Autodesk Inventor part; units mm, degrees
ref_plane "YZ Plane" through (0, 0, 0) normal (1, 0, 0) x (0, 1, 0)
ref_plane "XZ Plane" through (0, 0, 0) normal (0, 1, 0) x (-1, 0, 0)
ref_plane "XY Plane" through (0, 0, 0) normal (0, 0, 1) x (1, 0, 0)
sketch "Sketch2" plane through (0, 0, 0) normal (0, 0, 1) x (1, 0, 0)
  line L0 (-50.1541, 26.4593) -> (-15.1541, 26.4593)
  line L1 (-15.1541, 26.4593) -> (-15.1541, 29.4593)
  line L2 (-15.1541, 29.4593) -> (34.8459, 29.4593)
  line L3 (34.8459, 29.4593) -> (34.8459, 26.4593)
  line L4 (34.8459, 26.4593) -> (69.8459, 26.4593)
  line L5 (-50.1541, 26.4593) -> (-50.1541, -70.5407)
  line L6 (-50.1541, -70.5407) -> (-15.1541, -70.5407)
  line L7 (-15.1541, -70.5407) -> (-15.1541, -73.5407)
  line L8 (-15.1541, -73.5407) -> (34.8459, -73.5407)
  line L9 (34.8459, -73.5407) -> (34.8459, -70.5407)
  line L10 (34.8459, -70.5407) -> (69.8459, -70.5407)
  line L11 (69.8459, -70.5407) -> (69.8459, 26.4593)
  point P0 (0, 0)
  dimension "d0" = 3
  dimension "d1" = 50
  dimension "d2" = 35
  dimension "d3" = 35
  dimension "d4" = 97
  dimension "d5" = 97
  dimension "d6" = 3
  dimension "d7" = 35
  dimension "d8" = 50
  dimension "d9" = 35
extrude "Extrusion1" add sketch "Sketch2" along normal blind 3
sketch "Sketch3" plane through (0, 0, 3) normal (0, 0, 1) x (1, 0, 0)
  line L0 (34.8459, 29.4593) -> (-15.1541, 29.4593)
  line L1 (-15.1541, -73.5407) -> (34.8459, -73.5407)
  line L2 (-50.1541, 26.4593) -> (-50.1541, -70.5407)
  line L3 (69.8459, -70.5407) -> (69.8459, 26.4593)
  circle A0 centre (57.6459, 1.2193) radius 2
  circle A1 centre (57.6459, -45.5807) radius 2
  circle A2 centre (-28.3541, 1.2193) radius 2
  circle A3 centre (-28.3541, -45.5807) radius 2
  circle A4 centre (47.3959, -22.1807) radius 7
  line L4 (-16.4541, -2.7807) -> (34.4459, -2.7807)
  line L5 (34.4459, -2.7807) -> (34.4459, -42.7807)
  line L6 (34.4459, -42.7807) -> (-16.4541, -42.7807)
  line L7 (-16.4541, -42.7807) -> (-16.4541, -2.7807)
  line L8 (-38.3241, -7.0307) -> (-31.4241, -7.0307)
  line L9 (-31.4241, -7.0307) -> (-31.4241, -37.4307)
  line L10 (-31.4241, -37.4307) -> (-38.3241, -37.4307)
  line L11 (-38.3241, -37.4307) -> (-38.3241, -7.0307)
  point P0 (0, 0)
  dimension "d30" = 4
  dimension "d34" = 4
  dimension "d35" = 4
  dimension "d36" = 4
  dimension "d38" = 14
  dimension "d43" = 50.9
  dimension "d44" = 40
extrude "Extrusion2" cut sketch "Sketch3" against normal blind 10
sketch "Sketch4" plane through (-38.3241, -37.4307, 3) normal (1, 0, 0) x (0, 0, -1)
  line L0 (0, 30.4) -> (3, 30.4)
  line L1 (3, 30.4) -> (3, 0)
  line L2 (3, 0) -> (0, 0)
  line L3 (0, 0) -> (0, 30.4)
  point P0 (3, 37.4307)
extrude "Extrusion3" add sketch "Sketch4" along normal blind 10
sketch "Sketch5" plane through (0, 0, 3) normal (0, 0, 1) x (1, 0, 0)
  circle A0 centre (47.3959, -22.1807) radius 7
  circle A1 centre (47.3959, -22.1807) radius 8
  line L0 (-16.4541, -2.7807) -> (34.4459, -2.7807)
  line L1 (34.4459, -42.7807) -> (-16.4541, -42.7807)
  line L2 (35.4459, -43.7807) -> (-17.4541, -43.7807)
  line L3 (-17.4541, -43.7807) -> (-17.4541, -1.7807)
  line L4 (-17.4541, -1.7807) -> (35.4459, -1.7807)
  line L5 (35.4459, -1.7807) -> (35.4459, -43.7807)
  point P0 (0, 0)
extrude "Extrusion4" cut sketch "Sketch5" against normal blind 10 contours A0 | A1 | L2 L3 L4 L5
sketch "Sketch6" plane through (0, 0, 3) normal (0, 0, 1) x (1, 0, 0)
  point P0 (0, 0)
sketch "Sketch7" plane through (0, 0, 3) normal (0, 0, 1) x (1, 0, 0)
  point P0 (0, 0)
sketch "Sketch8" plane through (0, 0, 3) normal (0, 0, 1) x (1, 0, 0)
  point P0 (0, 0)
properties part number "Level2-3 (GLCD)"
The listing builds one solid part. Answer for the finished solid, in the listing's coordinates (mm). A direction names the side the tool comes from. Give positions to 0.01 mm unless a question says otherwise; leave off trailing zeros. Write each loop counter-clockwise with the first axis right and the second up, starting at its lowest first coordinate (ties: lowest second). Pieces come first, ordered by that corner, then holes.
1) Find the intervals of material crossed by L1, parallel to Y at x = 2, z = 0.2; L2, parallel to X at y = -38.5, z = 0.5; L3, parallel to Y at x = -17, z = 0.9, in increasing order.
2) A tool of negligible diameter and unlimited length cuts with its end or side. For faces 5 (the face through (52, -70.541, 1)), 6 (the face through (-15.154, 28, 1)), 7 (the face through (9, -43.781, 2)), from which of +Z, -Z, +X, -X, +Y, -Y can it reach the whole face along a straight path? Write none if from no direction.
3) Section C-C (z = 1.15) is taken. Write down the section's boundary in (x, y).
4) Given P1, Ø3.5, axis at x = 57.65, y = 1.22, coming from the +Z side (3 decimals); P2, Ø1.5, axis at y = -71.5, z = 1.5, coming from the -X side; P3, Ø0.9, axis at x = 60.5, z = 1.5, coming from the +Y side; P4, Ø1.5, axis at x = 36.5, z = 0.5, coming from the -Y side, each flat-ended and moving along its own axis, determine where each tip first touches the part or whether it passes through.
5) Section B-B (y = -40) is taken. Write down the section's boundary in (x, z).
6) Section D-D (x = -21) is taken. Write down the section's boundary in (y, z).
7) Section A-A (x = 7) is taken. Write down the section's boundary in (y, z), and give its area (3 significant figures).
8) For a pull along Y with two mould halves and no side action, classify faces 1 (the face through (34.846, -72, 1)), 2 (the face through (9, -1.781, 2)), 3 (the face through (52, 26.459, 1)), 4 (the face through (-33, -70.541, 1)) as pulls with the +Y half, pulls with the -Y half, needs draft (parallel to the pull), parting line crosses it, or undercut.
Response:
1. L1: y = -73.54 to -43.78, -1.78 to 29.46
1. L2: x = -50.15 to -17.45, 35.45 to 69.85
1. L3: y = -70.54 to -43.78, -1.78 to 26.46
2. face 5: +Z, -Z, +X, -Y
2. face 6: +Z, -Z, -X, +Y
2. face 7: +Z, -Z
3. outline: (-50.15, -70.54) - (-15.15, -70.54) - (-15.15, -73.54) - (34.85, -73.54) - (34.85, -70.54) - (69.85, -70.54) - (69.85, 26.46) - (34.85, 26.46) - (34.85, 29.46) - (-15.15, 29.46) - (-15.15, 26.46) - (-50.15, 26.46) - close; hole circle Ø4 at (-28.35, -45.58); hole circle Ø4 at (-28.35, 1.22); hole (-17.45, -43.78) - (35.45, -43.78) - (35.45, -1.78) - (-17.45, -1.78) - close; hole circle Ø16 at (47.4, -22.18); hole circle Ø4 at (57.65, -45.58); hole circle Ø4 at (57.65, 1.22)
4. P1: passes through
4. P2: stops at x = -15.15
4. P3: stops at y = 26.46
4. P4: stops at y = -70.54
5. outline: (-50.15, 0) - (-17.45, 0) - (-17.45, 3) - (-50.15, 3) - close; (35.45, 0) - (69.85, 0) - (69.85, 3) - (35.45, 3) - close
6. outline: (-70.54, 0) - (26.46, 0) - (26.46, 3) - (-70.54, 3) - close
7. outline: (-73.54, 0) - (-43.78, 0) - (-43.78, 3) - (-73.54, 3) - close; (-1.78, 0) - (29.46, 0) - (29.46, 3) - (-1.78, 3) - close
7. area: 183 mm2
8. face 1: needs draft
8. face 2: undercut
8. face 3: pulls with the +Y half
8. face 4: pulls with the -Y half
